Can you work these out from the model? Positions are in its coordinate system, mm. A direction names the side the tool comes from. Give positions to 0.01 mm unless a question says otherwise; leave off trailing zeros. Order: outer loops, then holes, each group sorted by start corner. A loop starts at its lowest first (then second) coordinate and runs counter-clockwise, first axis right, second up. Notation, with made-up numbers: (31.25, -3.75) - (61.25, -3.75) arc R19 cw to (61.25, 10.25) - close; hole circle Ø2 at (29, 73.5). An arc over 180 degrees is marked (long way). Return JSON: item names as keys, results as strings.
```python
from build123d import *

# Parameters (mm, degrees)
SKETCH_2_W   = 9.5
SKETCH_2_H   = 2.44
SKETCH_2_W_2 = 19.5
SKETCH_2_H_2 = 0.1


with BuildPart() as part:
    # 草图2 → 旋转1 (revolve)
    with BuildSketch(Plane.XY):
        with Locations((26.75, -1.22)):
            Rectangle(SKETCH_2_W, SKETCH_2_H)
        Polygon((24.665, -2.44), (22, -2.44), (22, -20.2), (22, -22.45), (24.665, -22.45), align=None)
        Polygon((22, -22.45), (22, -20.2), (19.5, -20.2), (19.5, -33.16), (19.5, -33.26), (22, -33.26), align=None)
        with Locations((9.75, -33.21)):
            Rectangle(SKETCH_2_W_2, SKETCH_2_H_2)
    revolve(axis=Axis((0, 6.935540238, 0), (0, -1, 0)))


solid = part.part
```
1. Suppose I cut it at D-D (y = -12). List the corners of the cut face in (x, z) for me (3 decimals), plus the area to 3 significant figures.
Checks:
{"outline": "circle Ø49.33 at (0, 0); hole circle Ø44 at (0, 0)", "area": "391 mm^2"}
2. Thinking about a two-plate mould opening in X: for faces 4 (the face through (19, -2.44, -16)), 5 (the face through (-4.769, -27.779, -21.477)), 6 (the face through (-2.539, -26.771, 19.334)), which applies, +X half, -X half, draft (parallel to the pull), parting line (faces both ways), or undercut?
Checks:
{"face 4": "draft", "face 5": "parting line", "face 6": "undercut"}
3. Suppose I cut it at C-C (z = 0). List the corners of the cut face in (x, y) for me (3 decimals).
Checks:
{"outline": "(-31.5, -2.44) - (-24.665, -2.44) - (-24.665, -22.45) - (-22, -22.45) - (-22, -33.26) - (22, -33.26) - (22, -22.45) - (24.665, -22.45) - (24.665, -2.44) - (31.5, -2.44) - (31.5, 0) - (22, 0) - (22, -20.2) - (19.5, -20.2) - (19.5, -33.16) - (-19.5, -33.16) - (-19.5, -20.2) - (-22, -20.2) - (-22, 0) - (-31.5, 0) - close"}
4. For pin 1 Ø6 at (y, z) = (-29.5, -23) entering from -X; pin 2 Ø19.5 at (x, z) = (0, 3.5) entering from +Y; pin 3 Ø12 at (x, y) = (16, -29.5) entering from -Z, each with a flat end and sliding along its axis, tell me the tip position at first contact or that it passes through.
Checks:
{"pin 1": "x = -9.17", "pin 2": "y = -33.16", "pin 3": "z = -19.6"}
5. On a 3-axis mill with a long thin cutter (end or side, diameter ignored), from which of +Z, -Z, +X, -X, +Y, -Y can I reach the whole of each face in a straight line? I mean faces 1 (the face through (-4.769, -10.241, -21.477)), 2 (the face through (-6.6, 0, 21.4)), 3 (the face through (22, -22.45, -4)). Say none if no direction works.
Checks:
{"face 1": "+Y", "face 2": "+Z, -Z, +X, -X, +Y", "face 3": "-Y"}
6. If I drill on L1, parallel to Z at x = 0, y = -26; L2, parallel to Z at x = 0, y = -6 (3 decimals); L3, parallel to Y at x = -16, z = -24, over which ranges is the centre line in solid material (lowest first)? Write a range as [from, to].
Checks:
{"L1": "[-22, -19.5], [19.5, 22]", "L2": "[-24.665, -22], [22, 24.665]", "L3": "[-2.44, 0]"}
7. Suppose I cut it at A-A (y = -28.5). List the corners of the cut face in (x, z) for me, plus the area to 3 significant figures.
Checks:
{"outline": "circle Ø44 at (0, 0); hole circle Ø39 at (0, 0)", "area": "326 mm^2"}
8. Suppose I cut it at B-B (x = 0). List the corners of the cut face in (y, z) for me (3 decimals).
Checks:
{"outline": "(-33.26, -22) - (-22.45, -22) - (-22.45, -24.665) - (-2.44, -24.665) - (-2.44, -31.5) - (0, -31.5) - (0, -22) - (-20.2, -22) - (-20.2, -19.5) - (-33.16, -19.5) - (-33.16, 19.5) - (-20.2, 19.5) - (-20.2, 22) - (0, 22) - (0, 31.5) - (-2.44, 31.5) - (-2.44, 24.665) - (-22.45, 24.665) - (-22.45, 22) - (-33.26, 22) - close"}
